Design review of the part built by this model. Coordinates are the model's own, in mm. Face numbers are marked on the shaded views. Round coordinates to 2 decimals unless told otherwise and drop trailing zeros. Write each loop counter-clockwise with the first axis right and the second up, starting at its lowest first coordinate (ties: lowest second). Pieces come first, ordered by that corner, then holes. Notation, with made-up numbers: (75, 41.5) - (94, 41.5) arc R35 cw to (94, 80.5) - close; hole circle Ø8 at (-20, -28). An arc over 180 degrees is marked (long way). Use one line per item in the form item = value.
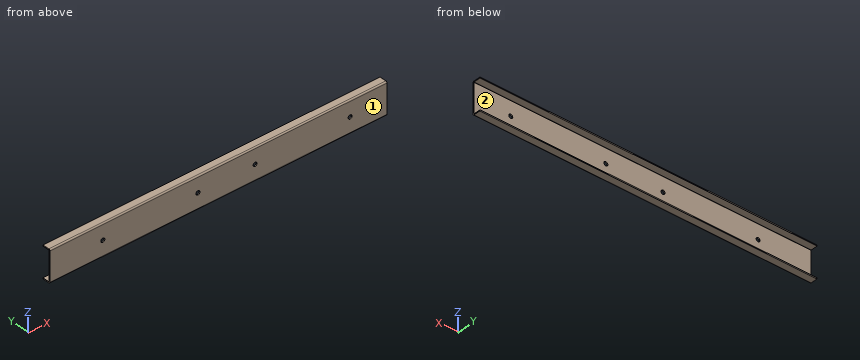
```python
from build123d import *

# Parameters (mm, degrees)
BASE_FLANGE1_DEPTH = 450
SKETCH6_R          = 2.667
CUT_EXTRUDE1_DEPTH = 1.4


# Sheet-metal steps are written as plain solids
with BuildPart() as part:
    # Sketch1 → Base-Flange1 (new body)
    with BuildSketch(Plane(origin=(0, 0, 0), x_dir=(0, 0, -1), z_dir=(1, 0, 0))):
        with BuildLine():
            Line((0, 10.75), (0, 1.65))
            ThreePointArc((0, 1.65), (0.483273811, 0.483273811), (1.65, 0))
            Line((1.65, 0), (40.35, 0))
            ThreePointArc((40.35, 0), (41.516726189, 0.483273811), (42, 1.65))
            Line((42, 1.65), (42, 10.75))
            Line((42, 10.75), (40.6, 10.75))
            Line((40.6, 10.75), (40.6, 1.65))
            ThreePointArc((40.6, 1.65), (40.526776695, 1.473223305), (40.35, 1.4))
            Line((40.35, 1.4), (1.65, 1.4))
            ThreePointArc((1.65, 1.4), (1.473223305, 1.473223305), (1.4, 1.65))
            Line((1.4, 1.65), (1.4, 10.75))
            Line((1.4, 10.75), (0, 10.75))
        make_face()
    extrude(amount=BASE_FLANGE1_DEPTH)

    # Sketch6 → Cut-Extrude1 (cut)
    with BuildSketch(Plane.XZ):
        with Locations(Location((400.7875, -21, 0), (0, 0, 270))):
            Circle(SKETCH6_R)
        with Locations(Location((273.7875, -21, 0), (0, 0, 270))):
            Circle(SKETCH6_R)
        with Locations(Location((197.5875, -21, 0), (0, 0, 270))):
            Circle(SKETCH6_R)
        with Locations(Location((70.5875, -21, 0), (0, 0, 270))):
            Circle(SKETCH6_R)
    extrude(amount=-CUT_EXTRUDE1_DEPTH, mode=Mode.SUBTRACT)


solid = part.part
```
Q1. For P1, Ø8.5, axis at x = 197.59, z = -21, coming from the +Y side, flat-tipped, find the tip position at first contact; note if it passes through.
Calculated:
P1 = 1.4
Q2. We need section B-B on z = -13. Write out the cut boundary in (x, y).
Calculated:
outline = (0, 0) - (450, 0) - (450, 1.4) - (0, 1.4) - close
Q3. We need section A-A on x = 218.5. Write out the cut boundary in (y, z), then the cut area to 3 significant figures.
Calculated:
outline = (0, -40.35) arc R1.65 ccw to (1.65, -42) - (10.75, -42) - (10.75, -40.6) - (1.65, -40.6) arc R0.25 cw to (1.4, -40.35) - (1.4, -1.65) arc R0.25 cw to (1.65, -1.4) - (10.75, -1.4) - (10.75, 0) - (1.65, 0) arc R1.65 ccw to (0, -1.65) - close
area = 83.8 mm2
Q4. Draft analysis for pull direction Z (two halves, no side actions). For the marked faces 1 and 2, state which applies: released by +Z, released by -Z, zero draft, split by the parting line, or undercut.
Calculated:
face_1 = zero draft
face_2 = undercut
Q5. To check wall thickness, follow line 1 along X through (y, z) = (1, -21); line 2 along Z through (x, y) = (371, 6); line 3 along Z through (x, y) = (94, 1.5). State the ranges of each line that lie inside material, in increasing order. Write a range as from..to.
Calculated:
line_1 = 0..67.92, 73.25..194.92, 200.25..271.12, 276.45..398.12, 403.45..450
line_2 = -42..-40.6, -1.4..0
line_3 = -41.99..-40.55, -1.45..-0.01
